Input: part model. Units: mm. Frame: model coordinates. A direction names the side the tool comes from. Give positions to 0.01 mm unless a question says otherwise; leave off trailing zeros. Write each loop counter-clockwise with the first axis right and the second up, starting at its lowest first coordinate (ties: lowest second). Pieces come first, ordered by that corner, then holes.
```python
from build123d import *

# Parameters (mm, degrees)
P_IDAT_VYSUNUT_M1_DEPTH = 3


with BuildPart() as part:
    # Skica1 → Přidat vysunutím1 (new body)
    with BuildSketch(Plane.XY):
        Polygon((35.098999138, -102.619674243), (25.567500119, -74.752232196), (28.406057565, -73.781360615), (24.522571242, -62.427130832), (21.684013796, -63.398002412), (10.357178687, -30.281498877), (13.195736133, -29.310627296), (9.311034651, -17.952844725), (6.472477205, -18.923716306), (0, 0), (65, 0), (66.054709497, -7.67410463), (63.082647903, -8.082577246), (64.716538365, -19.970823625), (67.68859996, -19.562351009), (68.743309457, -27.236455639), (73.306691143, -38.242479423), (70.535456643, -39.391504813), (75.131558201, -50.476442813), (77.902792701, -49.327417423), (82.466174387, -60.333441207), (98.069771345, -79.328299093), (95.751633165, -81.232566768), (103.368703864, -90.505119489), (105.686842044, -88.600851814), (121.290439003, -107.5957097), (101.634461089, -163.225221043), (89.098999138, -163.225221043), (89.098999138, -160.225221043), (77.098999138, -160.225221043), (77.098999138, -163.225221043), (62.098999138, -163.225221043), (62.098999138, -160.225221043), (50.098999138, -160.225221043), (50.098999138, -163.225221043), (35.098999138, -163.225221043), (35.098999138, -138.920221043), (38.098999138, -138.920221043), (38.098999138, -126.920221043), (35.098999138, -126.920221043), align=None)
        Polygon((53.581071902, -119.454548354), (62.452466829, -127.535287927), (64.472651723, -125.317439195), (55.601256796, -117.236699622), align=None, mode=Mode.SUBTRACT)
        Polygon((77.238125041, -141.003187216), (86.109519967, -149.083926789), (88.129704861, -146.866078058), (79.258309934, -138.785338484), align=None, mode=Mode.SUBTRACT)
    extrude(amount=P_IDAT_VYSUNUT_M1_DEPTH)


solid = part.part
```
Q1. Access query for faces 4 (the flat face through (3.28, -9.59, 1.48)), 5 (the flat face through (99.507, -85.804, 1.479)). Directions: +Z, -Z, +X, -X, +Y, -Y. A direction counts if a zero-diameter tool reaches every point of the face in a straight line with its end or side. Return the directions, or none.
Q2. Section A-A, the plane z = 0.8. Give the number of separate pieces and of enclosed holes in the cut face, then the cut area to 3 significant figures.
Q3. Section C-C, the plane y = -33.5. Return the cut outline in (x, z).
Q4. Material intervals for line 1 along X through (y, z) = (-122, 1.7); line 2 along Y through (x, z) = (51.5, 0.95); line 3 along X through (y, z) = (-50, 1.25), sorted ascending.
Q5. Section B-B, the plane y = -15.5. Return the cut outline in (x, z), then the cut area to 3 significant figures.
Q6. Mould query, pull axis Y, two halves, no side actions, for faces 1 (the flat face through (61, -80, 3)), 2 (the flat face through (70.99, -32.66, 1.48)), 3 (the flat face through (72.801, -44.856, 1.479)). Classes: +Y half, -Y half, draft (parallel to the pull), parting line (faces both ways), or undercut.
Q7. Pin query (flat end, axial travel): pin 1 (1.5 mm diameter, centred on y = -154.5, z = 1.5, fed in from -X); pin 2 (0.9 mm diameter, centred on x = 84.5, z = 1.5, fed in from -Y); pin 3 (1.5 mm diameter, centred on y = -134.5, z = 1.5, fed in from -X). Return the tip coordinate at first contact, or that it passes through.
Solutions:
1. face 4: +Z, -Z, -X, -Y
1. face 5: +Z, -Z
2. separate pieces: 1
2. enclosed holes: 2
2. area: 11,100 mm2
3. outline: (11.46, 0) - (71.34, 0) - (71.34, 3) - (11.46, 3) - close
4. line 1: x = 35.1 to 56.38, 60.83 to 116.2
4. line 2: y = -160.23 to 0
4. line 3: x = 17.1 to 74.93, 76.28 to 78.18
5. outline: (5.3, 0) - (64.1, 0) - (64.1, 3) - (5.3, 3) - close
5. area: 176 mm2
6. face 1: draft
6. face 2: +Y half
6. face 3: undercut
7. pin 1: stops at x = 35.1
7. pin 2: stops at y = -160.23
7. pin 3: stops at x = 38.1
